Autodesk Inventor part; units mm, degrees
ref_plane "YZ Plane" through (0, 0, 0) normal (1, 0, 0) x (0, 1, 0)
ref_plane "XZ Plane" through (0, 0, 0) normal (0, 1, 0) x (-1, 0, 0)
ref_plane "XY Plane" through (0, 0, 0) normal (0, 0, 1) x (1, 0, 0)
sketch "Sketch1" plane through (0, 0, 0) normal (0, 1, 0) x (-1, 0, 0)
  line L0 (-20, -11) -> (20, -11)
  line L1 (20, -11) -> (20, 11)
  line L2 (20, 11) -> (-20, 11)
  line L3 (-20, 11) -> (-20, -11)
  line L4 (-20, -11) -> (20, 11) construction
  line L5 (20, -11) -> (-20, 11) construction
  point P0 (0, 0)
  dimension "d0" = 22
  dimension "d1" = 40
extrude "Extrusion1" add sketch "Sketch1" along normal blind 12
sketch "Sketch2" plane through (0, 12, 0) normal (0, 1, 0) x (1, 0, 0)
  line L0 (20, -20) -> (-20, -20)
  line L1 (-20, -20) -> (-20, 20)
  line L2 (-20, 20) -> (20, 20)
  line L3 (20, 20) -> (20, -20)
  line L4 (20, -20) -> (-20, 20) construction
  line L5 (-20, -20) -> (20, 20) construction
  point P0 (0, 0)
  dimension "d4" = 40
  dimension "d5" = 40
extrude "Extrusion2" add sketch "Sketch2" along normal blind 5
sketch "Sketch3" plane through (0, 17, 0) normal (0, 1, 0) x (1, 0, 0)
  circle A0 centre (-15, -15) radius 3
  line L0 (-20, -20) -> (20, -20)
  line L1 (-20, 20) -> (-20, -20)
  circle A1 centre (15, -15) radius 3
  circle A2 centre (15, 15) radius 3
  circle A3 centre (-15, 15) radius 3
  line L2 (-20, 20) -> (20, 20)
  line L3 (20, -20) -> (20, 20)
  point P0 (0, 0)
  dimension "d8" = 6
  dimension "d9" = 5
  dimension "d10" = 5
  dimension "d11" = 6
  dimension "d12" = 6
  dimension "d13" = 6
  dimension "d14" = 5
  dimension "d15" = 5
  dimension "d16" = 5
  dimension "d17" = 5
  dimension "d18" = 5
  dimension "d19" = 5
extrude "Extrusion3" cut sketch "Sketch3" against normal blind 100 keep common part
sketch "Sketch4" plane through (-20, 0, 11) normal (0, 0, 1) x (1, 0, 0)
  circle A0 centre (10, 5) radius 3
  circle A1 centre (30, 5) radius 3
  line L0 (0, 0) -> (0, 12)
  line L1 (40, 0) -> (40, 12)
  line L2 (40, 0) -> (0, 0)
  point P0 (20, 0)
  dimension "d22" = 6
  dimension "d23" = 6
  dimension "d24" = 10
  dimension "d25" = 10
  dimension "d26" = 5
  dimension "d27" = 5
extrude "Extrusion4" cut sketch "Sketch4" against normal blind 100
properties part number "Conector"
Source: CAD feature listing. Evaluate the final solid. Frame: model axes, mm. A direction names the side the tool comes from. Coordinates: 2 decimals unless noted, no trailing zeros. Loops run counter-clockwise (first coordinate to the right, second up) from the corner with the lowest first, then second, coordinate; pieces in that order, holes last. Notation, with made-up numbers: (23.5, 89.5) -> (34.5, 89.5) arc R17 ccw to (34.5, 99.5) -> close; hole circle Ø6 at (43, 89.25). An arc over 180 degrees is marked (long way). Answer in a Markdown table with one row per item. Add a question column.
Q1. Contact query for flat-ended pins moving along their axis: pin 1 Ø4.5 at (x, z) = (0.5, 14) entering from -Y; pin 2 Ø1 at (x, y) = (11, 9.5) entering from +Z; pin 3 Ø9.5 at (x, y) = (7, 5.5) entering from -Z. Output: stop coordinate, or through.
Q2. Reachability of faces 1 (the face through (0, 12, -16)), 2 (the face through (0, 6, 11)), 3 (the face through (0, 0, 0)) from +Z, -Z, +X, -X, +Y, -Y: full face, straight path, thin tool, end or side. Return the list, or none.
Q3. Section C-C on x = 15. Return the cut outline in (y, z).
Q4. Pull-direction query (X, two-part tool) for faces 4 (the face through (-20, 10, 0)), 5 (the face through (0, 17, 0)), 6 (the face through (12.6, 14.5, -13.2)); classes: pulls with the +X half, pulls with the -X half, needs draft (parallel to the pull), parting line crosses it, or undercut.
Q5. Section A-A on x = 10. Return the cut outline in (y, z), and give its area (3 significant figures).
Q6. Section B-B on z = 15. Return the cut outline in (x, y).
Q7. Section D-D on z = 10. Return the cut outline in (x, y).
Q8. Ray query, line 1 along X through (y, z) = (4.75, -2); line 2 along Z through (x, y) = (-15, 15.35). Return the intervals inside material, ascending.
Computed values:
| question | item | result |
|---|---|---|
| 1 | pin 1 | stops at y = 12 |
| 1 | pin 2 | stops at z = 11 |
| 1 | pin 3 | stops at z = -11 |
| 2 | face 1 | -Z, +X, -X, -Y |
| 2 | face 2 | +Z, +X, -X, -Y |
| 2 | face 3 | +Z, -Z, +X, -X, -Y |
| 3 | outline | (0, -11) -> (12, -11) -> (12, -12) -> (17, -12) -> (17, 12) -> (12, 12) -> (12, 11) -> (0, 11) -> close; (12, -20) -> (17, -20) -> (17, -18) -> (12, -18) -> close; (12, 18) -> (17, 18) -> (17, 20) -> (12, 20) -> close |
| 4 | face 4 | pulls with the -X half |
| 4 | face 5 | needs draft |
| 4 | face 6 | undercut |
| 5 | outline | (0, -11) -> (2, -11) -> (2, 11) -> (0, 11) -> close; (8, -11) -> (12, -11) -> (12, -20) -> (17, -20) -> (17, 20) -> (12, 20) -> (12, 11) -> (8, 11) -> close |
| 5 | area | 332 mm^2 |
| 6 | outline | (-20, 12) -> (-18, 12) -> (-18, 17) -> (-20, 17) -> close; (-12, 12) -> (12, 12) -> (12, 17) -> (-12, 17) -> close; (18, 12) -> (20, 12) -> (20, 17) -> (18, 17) -> close |
| 7 | outline | (-20, 0) -> (20, 0) -> (20, 17) -> (-20, 17) -> close; hole circle Ø6 at (-10, 5); hole circle Ø6 at (10, 5) |
| 8 | line 1 | x = -20 to -12.99, -7.01 to 7.01, 12.99 to 20 |
| 8 | line 2 | z = -20 to -18, -12 to 12, 18 to 20 |
